Build history of the part. All positions in model axes, mm. A direction names the side the tool comes from. Give positions to 0.01 mm unless a question says otherwise; leave off trailing zeros. Write each loop counter-clockwise with the first axis right and the second up, starting at its lowest first coordinate (ties: lowest second). Pieces come first, ordered by that corner, then holes. Notation, with made-up numbers: M 11,-24 L 27,-24 A29 ccw 27,2 Z; hole C -7.5,68 d7. An arc over 180 degrees is marked long. Return JSON: item names as keys, results as strings. Group by question number.
Q1. Tool access for faces 4 (the flat face through (-5, 5, 0)), 5 (the flat face through (11, 2, 0)), 6 (the cylindrical face through (2.44, 40.16, 0.54)): list every direction of +Z, -Z, +X, -X, +Y, -Y with a clear straight run to the whole face (end or side of a thin tool).
Q2. Wall check: probe 1 along X at (y, z) = (1.55, 6); probe 2 along Z at (x, y) = (22.5, 7.5); probe 3 along X at (y, z) = (25.5, 2). Give the ranges that are in metal, low to high.
Q3. Band-saw the part on C-C, the plane z = -6. Give the cut face in (x, y), then the cut area to 3 significant figures.
Q4. Pull direction Z, two halves, no side cores. Call faces 1 (the cylindrical face through (6.751, 2.465, -3.615)), 2 (the flat face through (0, 2, 11)), 3 (the flat face through (60, 9, 0)): +Z half, -Z half, draft (parallel to the pull), parting line (faces both ways), or undercut.
Q5. Band-saw the part on B-B, the plane x = -6. Give the cut face in (y, z).
Q6. Band-saw the part on A-A, the plane z = 6. Give the cut face in (x, y).
Q7. Flat gauge pins, fed straight in: pin 1 Ø4.5 at (x, z) = (-6, 6) entering from -Y; pin 2 Ø8 at (x, z) = (-6, -6) entering from +Y; pin 3 Ø6.5 at (x, z) = (1, 4.5) entering from +Y; pin 4 Ø4 at (x, z) = (2, 10.5) entering from +Y. Where does each tip first touch, or does it go through?
Q8. Band-saw the part on D-D, the plane y = 50. Give the cut face in (x, z), then the cut area to 3 significant figures.
from build123d import *

# Parameters (mm, degrees)
SKETCH_1_W      = 22
SKETCH_1_H      = 22
SKETCH_1_R      = 2.5
EXTRUDE_2_DEPTH = 5
EXTRUDE_START   = 5
SKETCH_3_R      = 4
EXTRUDE_3_DEPTH = 4
SKETCH_5_R      = 2.5
EXTRUDE_4_DEPTH = 64
SKETCH_6_R      = 2.5
EXTRUDE_5_DEPTH = 60
SKETCH_7_R      = 2.5
EXTRUDE_6_DEPTH = 60


with BuildPart() as part:
    # 草图1 → 凸台-拉伸2 (new body)
    with BuildSketch(Plane(origin=(0, 0, 0), x_dir=(1, 0, 0), z_dir=(0, 1, 0))):
        Rectangle(SKETCH_1_W, SKETCH_1_H)
        with Locations(Location((-6, 6, 0), (0, 0, 270))):
            Circle(SKETCH_1_R, mode=Mode.SUBTRACT)
        with Locations(Location((6, 6, 0), (0, 0, 270))):
            Circle(SKETCH_1_R, mode=Mode.SUBTRACT)
        with Locations(Location((-6, -6, 0), (0, 0, 270))):
            Circle(SKETCH_1_R, mode=Mode.SUBTRACT)
        with Locations(Location((6, -6, 0), (0, 0, 270))):
            Circle(SKETCH_1_R, mode=Mode.SUBTRACT)
    extrude(amount=EXTRUDE_2_DEPTH)

    # 草图3 → 凸台-拉伸3 (add)
    with BuildSketch(Plane(origin=(0, 0, 0), x_dir=(1, 0, 0), z_dir=(0, 1, 0)).offset(EXTRUDE_START)):
        with Locations(Location((0, 0, 0), (0, 0, 90))):
            Circle(SKETCH_3_R)
    extrude(amount=EXTRUDE_3_DEPTH)

    # 草图4 → 旋转1 (revolve)
    with BuildSketch(Plane.XY):
        with BuildLine():
            Line((0, 13), (0, 5))
            ThreePointArc((0, 5), (4, 9), (0, 13))
        make_face()
    revolve(axis=Axis((0, -1000, 0), (0, 1, 0)))

    # 草图5 → 凸台-拉伸4 (add)
    with BuildSketch(Plane(origin=(0, 0, 0), x_dir=(1, 0, 0), z_dir=(0, 1, 0)).offset(EXTRUDE_START)):
        with Locations(Location((0, 0, 0), (0, 0, 90))):
            Circle(SKETCH_5_R)
    extrude(amount=EXTRUDE_4_DEPTH)

    # 草图6 → 凸台-拉伸5 (add)
    with BuildSketch(Plane.XY):
        with Locations((0, 9)):
            Circle(SKETCH_6_R)
    extrude(amount=EXTRUDE_5_DEPTH)

    # 草图7 → 凸台-拉伸6 (add)
    with BuildSketch(Plane(origin=(0, 0, 0), x_dir=(0, 0, -1), z_dir=(1, 0, 0))):
        with Locations((0.4387505, 9)):
            Circle(SKETCH_7_R)
    extrude(amount=EXTRUDE_6_DEPTH)


solid = part.part
From the geometry:
{
 "1": {"face 4": "none", "face 5": "+Z, -Z, +X, -Y", "face 6": "+Y"},
 "2": {"probe 1": "x = -11 to -8.5, -3.5 to 3.5, 8.5 to 11", "probe 2": "z = -2.44 to 1.56", "probe 3": "x = -1.5 to 1.5"},
 "3": {"outline": "M -11,0 L -8.5,0 L -8.5,5 L -11,5 Z; M -3.5,0 L 3.5,0 L 3.5,5 L -3.5,5 Z; M 8.5,0 L 11,0 L 11,5 L 8.5,5 Z", "area": "60.0 mm^2"},
 "4": {"face 1": "undercut", "face 2": "+Z half", "face 3": "draft"},
 "5": {"outline": "M 0,-11 L 5,-11 L 5,-8.5 L 0,-8.5 Z; M 0,-3.5 L 5,-3.5 L 5,3.5 L 0,3.5 Z; M 0,8.5 L 5,8.5 L 5,11 L 0,11 Z"},
 "6": {"outline": "M -11,0 L -8.5,0 L -8.5,5 L -11,5 Z; M -3.5,0 L 3.5,0 L 3.5,5 L -3.5,5 Z; C 0,9 d5; M 8.5,0 L 11,0 L 11,5 L 8.5,5 Z"},
 "7": {"pin 1": "passes through", "pin 2": "stops at y = 5", "pin 3": "stops at y = 69", "pin 4": "stops at y = 11.5"},
 "8": {"outline": "C 0,0 d5", "area": "19.6 mm^2"}
}
